Here's how the part is built. I have some questions about the finished solid (model axes, mm). Face numbers are marked on the shaded views. A direction names the side the tool comes from. Round coordinates to 2 decimals unless told otherwise and drop trailing zeros. Loops run counter-clockwise (first coordinate to the right, second up) from the corner with the lowest first, then second, coordinate; pieces in that order, holes last. Notation, with made-up numbers: M 31.25,33 L 90.25,33 A8 ccw 90.25,47 Z; hole C 80.5,60 d5. An arc over 180 degrees is marked long. Answer as a JSON object with one key per item and string values.
from build123d import *

# Parameters (mm, degrees)
SKETCH_1_R          = 2.75
EXTRUDE_1_DEPTH     = 5
SKETCH_2_R          = 2.5
CUT_EXTRUDE_1_DEPTH = 4.7
SKETCH_3_R          = 1.5
CUT_EXTRUDE_2_DEPTH = 4.7
EXTRUDE_START       = -2
SKETCH_4_R          = 1.25
EXTRUDE_3_DEPTH     = 2


with BuildPart() as part:
    # 草图1 → 凸台-拉伸1 (new body)
    with BuildSketch(Plane.XY):
        Circle(SKETCH_1_R)
    extrude(amount=EXTRUDE_1_DEPTH)

    # 草图2 → 切除-拉伸1 (cut)
    with BuildSketch(Plane(origin=(0, 0, 0), x_dir=(-1, 0, 0), z_dir=(0, 0, -1))):
        Circle(SKETCH_2_R)
    extrude(amount=-CUT_EXTRUDE_1_DEPTH, mode=Mode.SUBTRACT)

    # 草图3 → 切除-拉伸2 (cut)
    with BuildSketch(Plane.XY.offset(5)):
        Circle(SKETCH_3_R)
    extrude(amount=-CUT_EXTRUDE_2_DEPTH, mode=Mode.SUBTRACT)

    # 草图4 → 凸台-拉伸3 (add)
    with BuildSketch(Plane.XY.offset(5).offset(EXTRUDE_START)):
        with BuildLine():
            Line((29.941561076, 1.591009855), (0.106557862, 2.747934756))
            ThreePointArc((0.106557862, 2.747934756), (1.981859495, 1.906497558), (2.75, 0))
            ThreePointArc((2.75, 0), (1.982079977, -1.906268335), (0.10719348, -2.747910035))
            Line((0.10719348, -2.747910035), (29.94192829, -1.584084071))
            ThreePointArc((29.94192829, -1.584084071), (31.46874704, 0.003639496), (29.941561076, 1.591009855))
        make_face()
        with Locations((13.53, 0)):
            Circle(SKETCH_4_R, mode=Mode.SUBTRACT)
        with Locations((18.98, 0)):
            Circle(SKETCH_4_R, mode=Mode.SUBTRACT)
        with Locations((24.43, 0)):
            Circle(SKETCH_4_R, mode=Mode.SUBTRACT)
        with Locations((29.8799998, 0.003455751)):
            Circle(SKETCH_4_R, mode=Mode.SUBTRACT)
    extrude(amount=EXTRUDE_3_DEPTH)


solid = part.part
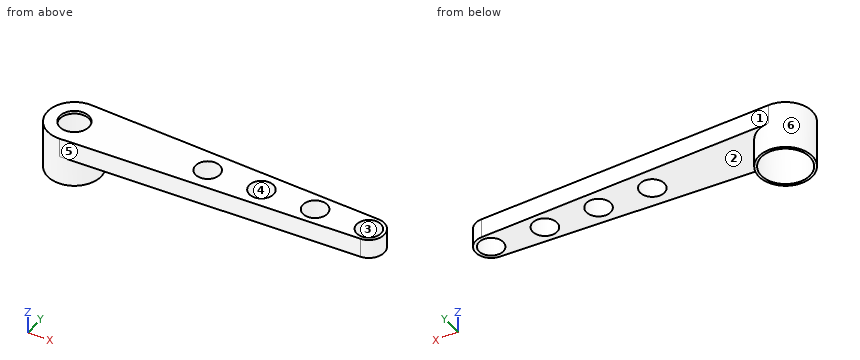
Item 1: I want a section at C-C on z = 1.5. List the corners of the cut face in (x, y) for me.
Solution:
{"outline": "C 0,0 d5.5; hole C 0,0 d5"}
Item 2: I want a section at B-B on x = 24.43. List the corners of the cut face in (y, z) for me.
Solution:
{"outline": "M -1.8,3 L -1.25,3 L -1.25,5 L -1.8,5 Z; M 1.25,3 L 1.8,3 L 1.8,5 L 1.25,5 Z"}
Item 3: If I drill on L1, parallel to Y at x = 29.88, z = 3.9; L2, parallel to X at y = 1.05, z = 4.85; L3, parallel to Y at x = 0, z = 3.75, over which ranges is the centre line in solid material (lowest first)? Write a range as from..to.
Solution:
{"L1": "y = -1.59..-1.25, 1.25..1.59", "L2": "x = -2.54..-1.07, 1.07..12.85, 14.21..18.3, 19.66..23.75, 25.11..29.2, 30.56..31.08", "L3": "y = -2.75..-2.5, 2.5..2.75"}
Item 4: For the marked faces 5 and 6, which set-ups out of +Z, -Z, +X, -X, +Y, -Y let a thin tool reach every point of the face, with its end or its side?
Solution:
{"face 5": "+Z, -Z, +X, -Y", "face 6": "-Z"}
Item 5: For P1, Ø1.5, axis at x = 24, z = 2, coming from the +Y side; P2, Ø2, axis at x = 14, y = -2, coming from the -Z side; P3, Ø2, axis at y = -0.5, z = 1.5, coming from the -X side, each with a flat end and sliding along its axis, tell me the tip position at first contact or that it passes through.
Solution:
{"P1": "passes through", "P2": "stops at z = 3", "P3": "stops at x = -2.75"}
Item 6: I want a section at D-D on x = 13.53. List the corners of the cut face in (y, z) for me, plus the area to 3 significant figures.
Solution:
{"outline": "M -2.22,3 L -1.25,3 L -1.25,5 L -2.22,5 Z; M 1.25,3 L 2.23,3 L 2.23,5 L 1.25,5 Z", "area": "3.90 mm2"}
Item 7: We'd pull the mould along Y, two halves only. Please class the marked faces 1, 2, 3 and 4: +Y half, -Y half, draft (parallel to the pull), parting line (faces both ways), or undercut.
Solution:
{"face 1": "+Y half", "face 2": "draft", "face 3": "undercut", "face 4": "undercut"}
Item 8: I want a section at A-A on y = 0.6. Count the separate pieces of the cut face and the enclosed holes in it, plus the area to 3 significant figures.
Solution:
{"separate pieces": "6", "enclosed holes": "0", "area": "43.0 mm2"}
